The model under review builds one solid part; all positions refer to its coordinate system, in mm. Face numbers are marked on the shaded views. A direction names the side the tool comes from. Give positions to 0.01 mm unless a question says otherwise; leave off trailing zeros. Loops run counter-clockwise (first coordinate to the right, second up) from the corner with the lowest first, then second, coordinate; pieces in that order, holes last. Notation, with made-up numbers: (-14, 6) - (-9, 6) arc R10 ccw to (-9, 22) - close; hole circle Ø2 at (75, 84). An arc over 180 degrees is marked (long way). Return JSON: item names as keys, results as strings. Group by question number.
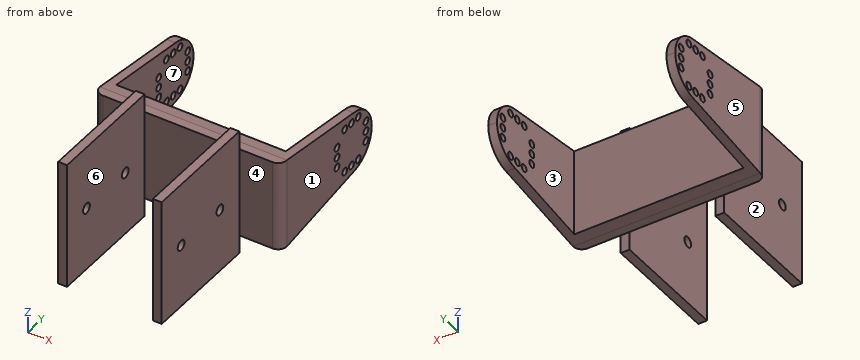
from build123d import *

# Parameters (mm, degrees)
SKETCH2_W           = 63.52
SKETCH2_H           = 30.59
BOSS_EXTRUDE1_DEPTH = 7
SKETCH3_W           = 3
SKETCH3_H           = 30.59
BOSS_EXTRUDE2_DEPTH = 40
FILLET2_R           = 3
SKETCH4_R           = 1.25
CUT_EXTRUDE2_DEPTH  = 70
SKETCH14_W          = 3
SKETCH14_H          = 43.15
BOSS_EXTRUDE5_DEPTH = 40.2
SKETCH15_R          = 1.75
CUT_EXTRUDE9_DEPTH  = 40


with BuildPart() as part:
    # Sketch2 → Boss-Extrude1 (new body)
    with BuildSketch(Plane(origin=(0, 0, 0), x_dir=(1, 0, 0), z_dir=(0, 1, 0))):
        with Locations((-20.26308022, 14.924105874)):
            Rectangle(SKETCH2_W, SKETCH2_H)
    extrude(amount=BOSS_EXTRUDE1_DEPTH)

    # Sketch3 → Boss-Extrude2 (add)
    with BuildSketch(Plane(origin=(0, 7, 0), x_dir=(1, 0, 0), z_dir=(0, 1, 0))):
        with Locations((-50.52308022, 14.924105874)):
            Rectangle(SKETCH3_W, SKETCH3_H)
        with Locations((9.99691978, 14.924105874)):
            Rectangle(SKETCH3_W, SKETCH3_H)
    extrude(amount=BOSS_EXTRUDE2_DEPTH)

    # Fillet2
    fillet2_edges = [part.edges().sort_by_distance(p)[0] for p in [
        (11.49691978, 0, -14.924105874),
        (-52.02308022, 0, -14.924105874),
    ]]
    fillet(fillet2_edges, radius=FILLET2_R)

    # Sketch4 → Cut-Extrude2 (cut)
    with BuildSketch(Plane.ZY.offset(52.02308022)):
        with BuildLine():
            ThreePointArc((-25.359340899, 37.664418298), (-21.924948962, 44.325483759), (-14.924105874, 47))
            Line((-14.924105874, 47), (-30.219105874, 47))
            Line((-30.219105874, 47), (-30.219105874, 3))
            Line((-30.219105874, 3), (-25.359340899, 37.664418298))
        make_face()
        with BuildLine():
            Line((0.370894126, 47), (-14.924105874, 47))
            ThreePointArc((-14.924105874, 47), (-7.923262787, 44.325483759), (-4.488870849, 37.664418298))
            Line((-4.488870849, 37.664418298), (0.370894126, 3))
            Line((0.370894126, 3), (0.370894126, 47))
        make_face()
        with Locations((-7.424105874, 36.5)):
            Circle(SKETCH4_R)
        with Locations((-7.424105874, 40)):
            Circle(SKETCH4_R)
        with Locations((-7.424105874, 33)):
            Circle(SKETCH4_R)
        with Locations((-14.924105874, 29)):
            Circle(SKETCH4_R)
        with Locations((-11.424105874, 29)):
            Circle(SKETCH4_R)
        with Locations((-18.424105874, 29)):
            Circle(SKETCH4_R)
        with Locations((-22.424105874, 36.5)):
            Circle(SKETCH4_R)
        with Locations((-22.424105874, 40)):
            Circle(SKETCH4_R)
        with Locations((-22.424105874, 33)):
            Circle(SKETCH4_R)
        with Locations((-11.424105874, 44)):
            Circle(SKETCH4_R)
        with Locations((-18.424105874, 44)):
            Circle(SKETCH4_R)
        with Locations((-14.924105874, 44)):
            Circle(SKETCH4_R)
    extrude(amount=-CUT_EXTRUDE2_DEPTH, mode=Mode.SUBTRACT)

    # Sketch14 → Boss-Extrude5 (add)
    with BuildSketch(Plane.XZ):
        with Locations((-36.32808022, -14.924105874)):
            Rectangle(SKETCH14_W, SKETCH14_H)
        with Locations((-4.19808022, -14.924105874)):
            Rectangle(SKETCH14_W, SKETCH14_H)
    extrude(amount=BOSS_EXTRUDE5_DEPTH)

    # Sketch15 → Cut-Extrude9 (cut)
    with BuildSketch(Plane.ZY.offset(37.82808022)):
        with Locations((-14.924105874, -30.15)):
            Circle(SKETCH15_R)
        with Locations((-14.924105874, -10.05)):
            Circle(SKETCH15_R)
    extrude(amount=-CUT_EXTRUDE9_DEPTH, mode=Mode.SUBTRACT)


solid = part.part
Item 1: For P1, Ø3, axis at x = -26.5, z = -29, coming from the +Y side; P2, Ø3, axis at y = 29, z = -14.92, coming from the -X side; P3, Ø3.5, axis at x = -37, z = 5, coming from the +Y side; P4, Ø5, axis at x = 0, z = -3, coming from the -Y side, all flat-tipped, find the tip position at first contact; note any pin that passes through.
Item 2: Take a section at C-C (x = -47.5). State the section outline as (y, z) points, then the cut area to 3 significant figures.
Item 3: Take a section at D-D (y = 29). State how many separate pieces and enclosed holes the cut face has, then the cut area to 3 significant figures.
Item 4: Take a section at B-B (y = -30.15). State the section outline as (x, z) points.
Item 5: Take a section at A-A (y = -1.5). State the section outline as (x, z) points, then the cut area to 3 significant figures.
Item 6: For L1, parallel to X at y = -32, z = -30; L2, parallel to X at y = 7.5, z = -29; L3, parallel to Y at x = -46, z = -27, list the stretches that pass through material, from the lowest coordinate up. Write a range as from..to.
Item 7: Mouldability with a two-part tool opening along X and no side actions: class the marked faces 1, 2 and 3 as +X half, -X half, draft (parallel to the pull), parting line (faces both ways), or undercut.
Item 8: Tool access review of the marked faces 4, 5, 6 and 7: name each direction out of +Z, -Z, +X, -X, +Y, -Y from which nothing blocks a thin tool from reaching the whole face with its end or side.
Check sheet entries:
{
 "1": {"P1": "stops at y = 7", "P2": "stops at x = -52.02", "P3": "stops at y = 0", "P4": "stops at y = 0"},
 "2": {"outline": "(0, -30.22) - (3, -30.22) - (7, -29.66) - (7, -0.19) - (3, 0.37) - (0, 0.37) - close", "area": "212 mm^2"},
 "3": {"separate pieces": "8", "enclosed holes": "0", "area": "94.8 mm^2"},
 "4": {"outline": "(-37.83, -36.5) - (-34.83, -36.5) - (-34.83, -16.67) - (-37.83, -16.67) - close; (-37.83, -13.17) - (-34.83, -13.17) - (-34.83, 6.65) - (-37.83, 6.65) - close; (-5.7, -36.5) - (-2.7, -36.5) - (-2.7, -16.67) - (-5.7, -16.67) - close; (-5.7, -13.17) - (-2.7, -13.17) - (-2.7, 6.65) - (-5.7, 6.65) - close"},
 "5": {"outline": "(-37.83, -36.5) - (-34.83, -36.5) - (-34.83, 6.65) - (-37.83, 6.65) - close; (-5.7, -36.5) - (-2.7, -36.5) - (-2.7, 6.65) - (-5.7, 6.65) - close", "area": "259 mm^2"},
 "6": {"L1": "x = -37.83..-34.83, -5.7..-2.7", "L2": "x = -52.02..-49.02, 8.5..11.5", "L3": "y = 0..7"},
 "7": {"face 1": "+X half", "face 2": "-X half", "face 3": "undercut"},
 "8": {"face 4": "+Z, -Z, +X, -Y", "face 5": "+Z, -Z, -X, +Y, -Y", "face 6": "+Z, -Z, -Y", "face 7": "+Z, -Z, +Y"}
}
